Job drawing, mm, ordinate dimensions from the low corner. One solid piece. Round coordinates to 2 decimals unless told otherwise and drop trailing zeros. Order: outer loops, then holes, each group sorted by start corner. A loop starts at its lowest first (then second) coordinate and runs counter-clockwise, first axis right, second up. Notation, with made-up numbers: (20, -2.5) - (64, -2.5) arc R14 cw to (64, 8.5) - close; hole circle Ø11 at (50.25, 29.25). An arc over 180 degrees is marked (long way). Use one line per item in the form item = value. Start each with the question number.
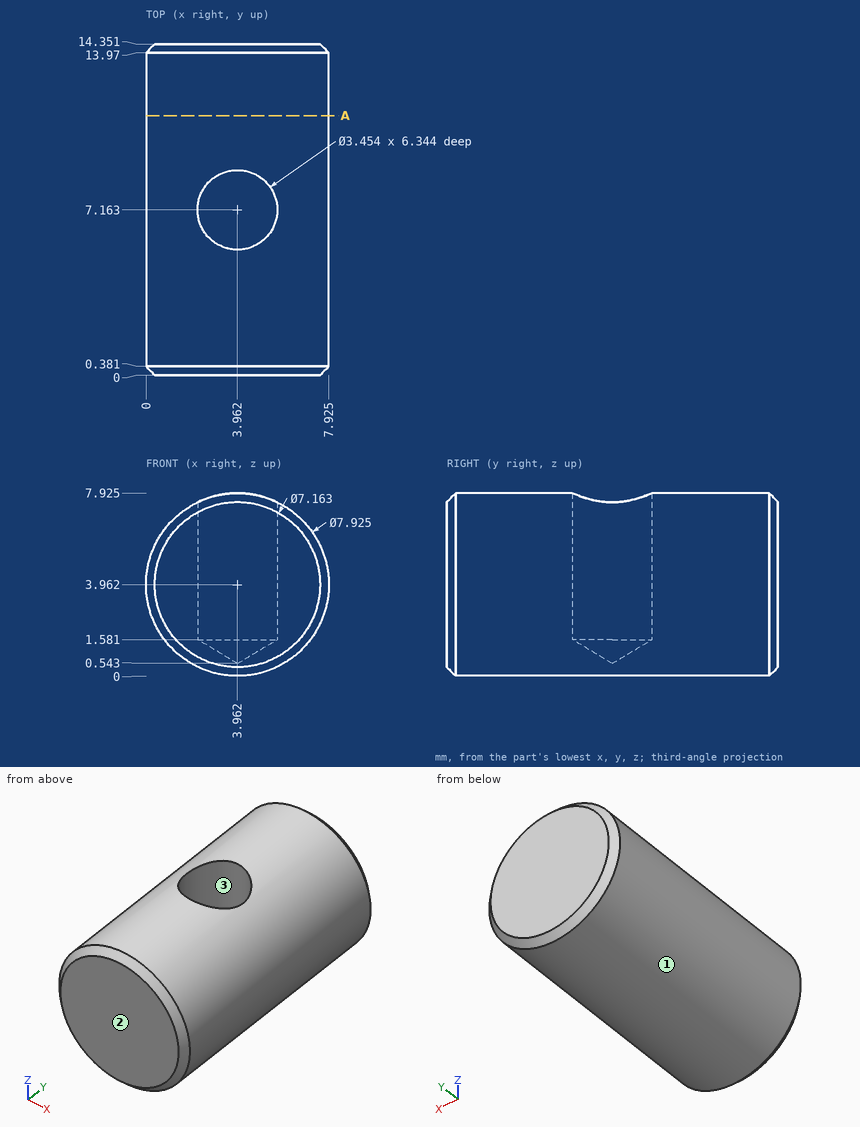
(1) Wall check: line 1 (X direction, y = 6, z = 4.75) (1 decimal); line 2 (X direction, y = 6, z = 2.5) (1 decimal); line 3 (X direction, y = 1.25, z = 5.75) (1 decimal). Give the ranges that are in metal, low to high. Write a range as [from, to].
(2) Flat gauge pin, fed straight in: P1, Ø1, axis at x = 7, y = 7, coming from the +Z side (1 decimal). Where does the tip first touch, or does it go through?
(3) Slice it at A-A (y = 11.25). Give the cut face in (x, z) (1 decimal), and give its area (3 significant figures).
(4) Mould opens along X. For the marked faces 1, 2 and 3 say: pulls with the +X half, pulls with the -X half, needs draft (parallel to the pull), parting line crosses it, or undercut.
Results list:
q1.line_1 = [0.1, 2.7], [5.2, 7.8]
q1.line_2 = [0.3, 2.7], [5.2, 7.6]
q1.line_3 = [0.4, 7.5]
q2.P1 = 7
q3.outline = circle Ø7.9 at (4, 4)
q3.area = 49.3 mm²
q4.face_1 = parting line crosses it
q4.face_2 = needs draft
q4.face_3 = undercut
